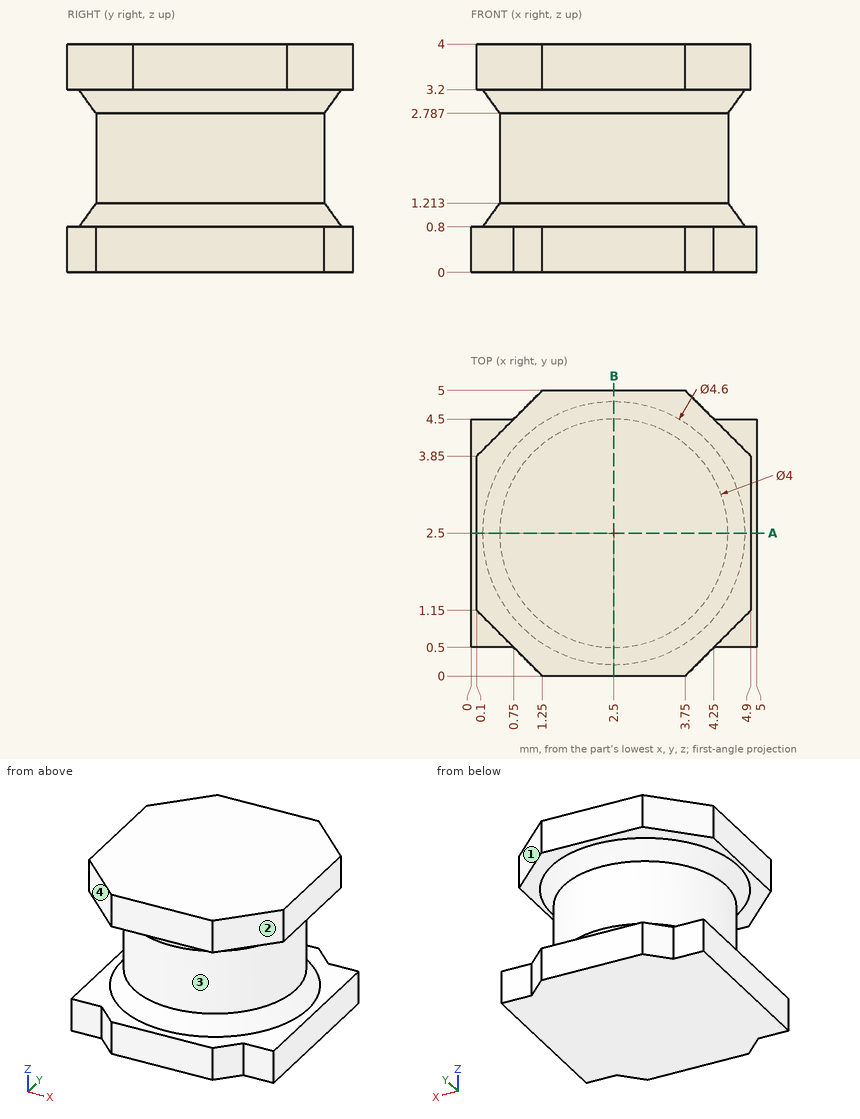
Could you check a few things on this drawing? It's one solid part, dimensions in mm from its lowest x, y, z. A direction names the side the tool comes from. Coordinates: 2 decimals unless noted, no trailing zeros. Write each loop counter-clockwise with the first axis right and the second up, starting at its lowest first coordinate (ties: lowest second). Pieces come first, ordered by that corner, then holes.
Q1. For P1, Ø0.9, axis at y = 2.5, z = 3.5, coming from the -X side; P2, Ø0.6, axis at x = 0.5, z = 0.5, coming from the +Y side; P3, Ø0.6, axis at y = 2, z = 3.5, coming from the +X side, each with a flat end and sliding along its axis, tell me the tip position at first contact or that it passes through.
Results found:
P1: stops at x = 0.1
P2: stops at y = 4.55
P3: stops at x = 4.9
Q2. Imagine slicing it at A-A, the plane y = 2.5. List the corners of the cut face in (x, z) for me, plus the area to 3 significant figures.
Results found:
outline: (0, 0) - (5, 0) - (5, 0.8) - (4.8, 0.8) - (4.5, 1.21) - (4.5, 2.79) - (4.8, 3.2) - (4.9, 3.2) - (4.9, 4) - (0.1, 4) - (0.1, 3.2) - (0.2, 3.2) - (0.5, 2.79) - (0.5, 1.21) - (0.2, 0.8) - (0, 0.8) - close
area: 17.7 mm2
Q3. Which directions (+Z, -Z, +X, -X, +Y, -Y) give clear straight access to the entire face, cutting with the end or side of a thin tool? Please do the marked faces 1, 2, 3 and 4.
Results found:
face 1: +Z, +X, +Y
face 2: +Z, +X, -Y
face 3: none
face 4: +Z, -X, -Y
Q4. Imagine slicing it at B-B, the plane x = 2.5. List the corners of the cut face in (y, z) for me.
Results found:
outline: (0, 0) - (5, 0) - (5, 0.8) - (4.8, 0.8) - (4.5, 1.21) - (4.5, 2.79) - (4.8, 3.2) - (5, 3.2) - (5, 4) - (0, 4) - (0, 3.2) - (0.2, 3.2) - (0.5, 2.79) - (0.5, 1.21) - (0.2, 0.8) - (0, 0.8) - close
Q5. Please list where these lines run through material, in increasing order: L1, parallel to Z at x = 4.2, y = 4.15; L2, parallel to Z at x = 1.55, y = 0.5; L3, parallel to X at y = 3.95, z = 3.1.
Results found:
L1: z = 0 to 0.8, 3.2 to 4
L2: z = 0 to 0.92, 3.08 to 4
L3: x = 0.81 to 4.19
